from build123d import *

# Parameters (mm, degrees)
F1_DEPTH      = 25
F3_W          = 2.0907083526
F3_H          = 4.3556410819
F4_DEPTH      = 59.0010001
F4_DEPTH_BACK = 25


with BuildPart() as f1:
    # F0 (on Top) → F1 (new body)
    with BuildSketch(Plane.XY):
        with BuildLine():
            Line((28, 0), (0, 0))
            Line((0, 0), (-28, 0))
            ThreePointArc((-28, 0), (-29.4142135624, 0.5857864376), (-30, 2))
            Line((-30, 2), (-30, 5))
            ThreePointArc((-30, 5), (-29.4142135624, 6.4142135624), (-28, 7))
            Line((-28, 7), (-21, 7))
            ThreePointArc((-21, 7), (-20.2928932188, 7.2928932188), (-20, 8))
            Line((-20, 8), (-20, 10))
            ThreePointArc((-20, 10), (-20.2928932188, 10.7071067812), (-21, 11))
            Line((-21, 11), (-28, 11))
            ThreePointArc((-28, 11), (-32.2426406871, 9.2426406871), (-34, 5))
            Line((-34, 5), (-34, 2))
            ThreePointArc((-34, 2), (-33.2295778289, -0.9413459047), (-31.116161423, -3.1273324435))
            add(Edge.make_bspline(
                [(-20.2002647828, -31.033764074), (-20.2216697913, -27.1145849984), (-17.4005191837, -17.4814529394), (-24.9095102489, -10.2786252936), (-27.0259722507, -5.2164699757), (-31.116161423, -3.1273324435)],
                knots=[0.0299386357, 0.0299386357, 0.0299386357, 0.0299386357, 0.374142378, 0.6819001297, 1, 1, 1, 1], degree=3))
            ThreePointArc((-20.2002647828, -31.033764074), (-19.9054528943, -31.7373376424), (-19.200279697, -32.0283025503))
            Line((-19.200279697, -32.0283025503), (-18.4729532019, -32.0283025503))
            ThreePointArc((-18.4729532019, -32.0283025503), (-17.7852228965, -31.7542688216), (-17.474415191, -31.0823566044))
            ThreePointArc((-17.474415191, -31.0823566044), (-12.0352803446, -19.323892803), (0, -14.5283025503))
            ThreePointArc((0, -14.5283025503), (12.0352803446, -19.323892803), (17.474415191, -31.0823566044))
            ThreePointArc((17.474415191, -31.0823566044), (17.7852228965, -31.7542688216), (18.4729532019, -32.0283025503))
            Line((18.4729532019, -32.0283025503), (19.200279697, -32.0283025503))
            ThreePointArc((19.200279697, -32.0283025503), (19.9054528943, -31.7373376424), (20.2002647828, -31.033764074))
            add(Edge.make_bspline(
                [(20.2002647828, -31.033764074), (20.2216697913, -27.1145849984), (17.4005191837, -17.4814529394), (24.9095102489, -10.2786252936), (27.0259722507, -5.2164699757), (31.116161423, -3.1273324435)],
                knots=[0.0299386357, 0.0299386357, 0.0299386357, 0.0299386357, 0.374142378, 0.6819001297, 1, 1, 1, 1], degree=3))
            ThreePointArc((31.116161423, -3.1273324435), (33.2295778289, -0.9413459047), (34, 2))
            Line((34, 2), (34, 5))
            ThreePointArc((34, 5), (32.2426406871, 9.2426406871), (28, 11))
            Line((28, 11), (21, 11))
            ThreePointArc((21, 11), (20.2928932188, 10.7071067812), (20, 10))
            Line((20, 10), (20, 8))
            ThreePointArc((20, 8), (20.2928932188, 7.2928932188), (21, 7))
            Line((21, 7), (28, 7))
            ThreePointArc((28, 7), (29.4142135624, 6.4142135624), (30, 5))
            Line((30, 5), (30, 2))
            ThreePointArc((30, 2), (29.4142135624, 0.5857864376), (28, 0))
        make_face()
        Polygon((-6, -2.6120110326), (0, -2.6120110326), (6, -2.6120110326), (6, -5.8120110326), (-6, -5.8120110326), align=None, mode=Mode.SUBTRACT)
    extrude(amount=F1_DEPTH)

    # F3 (on offset) → F4 (cut, two sides)
    with BuildSketch(Plane.YZ.offset(25)) as f4_sk:
        with Locations((-9.738416411, 19.4626431912)):
            Rectangle(F3_W, F3_H)
        with Locations((-9.7166006453, 6.0226437636)):
            Rectangle(F3_W, F3_H)
    extrude(amount=-F4_DEPTH, mode=Mode.SUBTRACT)
    extrude(f4_sk.sketch, amount=F4_DEPTH_BACK, mode=Mode.SUBTRACT)


solid = f1.part
CAD build for the part. Positions are in the model's coordinates, mm. A direction names the side the tool comes from. Give positions to 0.01 mm unless a question says otherwise; leave off trailing zeros. Order: outer loops, then holes, each group sorted by start corner. A loop starts at its lowest first (then second) coordinate and runs counter-clockwise, first axis right, second up. Notation, with made-up numbers: (44.25, 4) - (56.25, 4) arc R25 cw to (56.25, 21) - close; hole circle Ø11 at (-17.75, 56.25). An arc over 180 degrees is marked (long way). Write each question's results on one line, items separated by ' | '.
1. Saw through at B-B on x = -13.5. List the corners of the cut face in (y, z).
Calculated:
outline: (-20.89, 0) - (0, 0) - (0, 25) - (-20.89, 25) - close; hole (-10.78, 17.28) - (-8.69, 17.28) - (-8.69, 21.64) - (-10.78, 21.64) - close; hole (-10.76, 3.84) - (-8.67, 3.84) - (-8.67, 8.2) - (-10.76, 8.2) - close
2. Saw through at A-A on y = 4. List the corners of the cut face in (x, z).
Calculated:
outline: (-34, 0) - (-30, 0) - (-30, 25) - (-34, 25) - close; (30, 0) - (34, 0) - (34, 25) - (30, 25) - close
3. 3-axis set-ups, long thin cutter, end or side, ignore diameter. For faces 1 (the face through (6, -4, 12)), 2 (the face through (0, -8.693, 19)), 3 (the face through (20, 9, 12)): which of +Z, -Z, +X, -X, +Y, -Y reach the whole face in a straight line?
Calculated:
face 1: +Z, -Z | face 2: +X, -X | face 3: +Z, -Z, +Y
4. Probe L1, parallel to Y at x = 0.5, z = 9.5; L2, parallel to Y at x = 4, z = 6.25; L3, parallel to X at y = -29.5, z = 22. List the from-to ranges inside material, lowest first. Write a range as from..to.
Calculated:
L1: y = -14.54..-5.81, -2.61..0 | L2: y = -14.99..-10.76, -8.67..-5.81, -2.61..0 | L3: x = -20.14..-17.32, 17.32..20.14
5. Pin check, flat tips, straight feed: pin 1 (7.5 mm diameter, centred on x = 8.5, z = 10.5, fed in from +Y); pin 2 (1.6 mm diameter, centred on y = -4, z = 18, fed in from -X); pin 3 (2 mm diameter, centred on x = -11, z = 19.5, fed in from -Y); pin 4 (1.5 mm diameter, centred on x = 14, y = -24, fed in from -Z). Stop position of each tip, or through.
Calculated:
pin 1: stops at y = 0 | pin 2: stops at x = -30.98 | pin 3: stops at y = -19.29 | pin 4: passes through
6. Pull direction Z, two halves, no side cores. Call faces 4 (the face through (0, 0, 12)), 5 (the face through (0, -10, 3.845)), 6 (the face through (0, -1, 0)), 7 (the face through (0, -10.762, 6)): released by +Z, released by -Z, zero draft, split by the parting line, or undercut.
Calculated:
face 4: zero draft | face 5: undercut | face 6: released by -Z | face 7: undercut
7. Saw through at D-D on x = 11. List the corners of the cut face in (y, z).
Calculated:
outline: (-18.42, 0) - (0, 0) - (0, 25) - (-18.42, 25) - close; hole (-10.78, 17.28) - (-8.69, 17.28) - (-8.69, 21.64) - (-10.78, 21.64) - close; hole (-10.76, 3.84) - (-8.67, 3.84) - (-8.67, 8.2) - (-10.76, 8.2) - close
8. Saw through at C-C on x = 23. Count the separate pieces of the cut face and the enclosed holes in it, and give its area (3 significant figures).
Calculated:
separate pieces: 2 | enclosed holes: 2 | area: 376 mm2
